CAD build for the part. Positions are in the model's coordinates, mm. Face numbers are marked on the shaded views. A direction names the side the tool comes from. Give positions to 0.01 mm unless a question says otherwise; leave off trailing zeros. Loops run counter-clockwise (first coordinate to the right, second up) from the corner with the lowest first, then second, coordinate; pieces in that order, holes last. Notation, with made-up numbers: (36.25, 85) - (90.25, 85) arc R26 ccw to (90.25, 102) - close; hole circle Ø10 at (-11, 87). An arc over 180 degrees is marked (long way). Return JSON: item names as keys, results as strings.
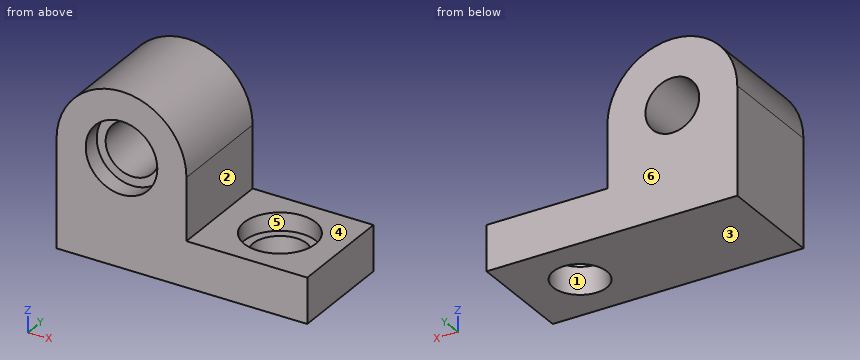
from build123d import *

# Parameters (mm, degrees)
F0_R     = 25.4
F0_R_2   = 19.05
F1_DEPTH = 76.2
F2_DEPTH = 12.7
F3_R     = 19.05
F4_DEPTH = 32.133529
F3_R_2   = 25.4
F5_DEPTH = 12.7


with BuildPart() as f1:
    # F0 (on Front) → F1 (new body)
    with BuildSketch(Plane.XZ):
        with BuildLine():
            Line((0, 76.2), (0, 0))
            Line((0, 0), (177.8, 0))
            Line((177.8, 0), (177.8, 32.132529))
            Line((177.8, 32.132529), (92.11325, 32.132529))
            Line((92.11325, 32.132529), (92.11325, 76.2))
            ThreePointArc((92.11325, 76.2), (46.056625, 122.256625), (0, 76.2))
        make_face()
        with Locations((46.056625, 76.2)):
            Circle(F0_R, mode=Mode.SUBTRACT)
        with Locations((46.056625, 76.2)):
            Circle(F0_R)
        with Locations((46.056625, 76.2)):
            Circle(F0_R_2, mode=Mode.SUBTRACT)
    extrude(amount=-F1_DEPTH)

    # F0 (on Front) → F2 (cut)
    with BuildSketch(Plane.XZ):
        with Locations((46.056625, 76.2)):
            Circle(F0_R)
        with Locations((46.056625, 76.2)):
            Circle(F0_R_2, mode=Mode.SUBTRACT)
    extrude(amount=-F2_DEPTH, mode=Mode.SUBTRACT)

    # F3 (on face) → F4 (cut, through all)
    with BuildSketch(Plane.XY.offset(32.132529)):
        with Locations((134.956625, 38.1)):
            Circle(F3_R)
    extrude(amount=-F4_DEPTH, mode=Mode.SUBTRACT)

    # F3 (on face) → F5 (cut)
    with BuildSketch(Plane.XY.offset(32.132529)):
        with Locations((134.956625, 38.1)):
            Circle(F3_R_2)
        with Locations((134.956625, 38.1)):
            Circle(F3_R, mode=Mode.SUBTRACT)
    extrude(amount=-F5_DEPTH, mode=Mode.SUBTRACT)


solid = f1.part
1. Pull direction X, two halves, no side cores. Call the marked faces 1, 2 and 3: +X half, -X half, draft (parallel to the pull), parting line (faces both ways), or undercut.
Values follow:
{"face 1": "undercut", "face 2": "+X half", "face 3": "draft"}
2. Cut at B-B, the plane x = 123. Write the cut outline in (y, z), plus the area to 3 significant figures.
Values follow:
{"outline": "(0, 0) - (23.27, 0) - (23.27, 19.43) - (15.69, 19.43) - (15.69, 32.13) - (0, 32.13) - close; (52.93, 0) - (76.2, 0) - (76.2, 32.13) - (60.51, 32.13) - (60.51, 19.43) - (52.93, 19.43) - close", "area": "1,300 mm²"}
3. Cut at D-D, the plane z = 63.5. Write the cut outline in (x, y).
Values follow:
{"outline": "(0, 0) - (24.06, 0) - (24.06, 12.7) - (31.86, 12.7) - (31.86, 76.2) - (0, 76.2) - close; (60.26, 12.7) - (68.05, 12.7) - (68.05, 0) - (92.11, 0) - (92.11, 76.2) - (60.26, 76.2) - close"}
4. Drill centre lines: probe 1 along X at (y, z) = (69, 75.5); probe 2 along Z at (x, y) = (45, 5); probe 3 along Z at (x, y) = (119, 23). Where is each one in solid material? Low to high.
Values follow:
{"probe 1": "x = 0 to 27.02, 65.09 to 92.11", "probe 2": "z = 0 to 50.82, 101.58 to 122.24", "probe 3": "z = 0 to 19.43"}
5. Drop flat-ended pins along their axis: P1, Ø1.5, axis at x = 58, z = 88, coming from the +Y side; P2, Ø1.5, axis at y = 14.5, z = 58.5, coming from the +X side; P3, Ø1, axis at y = 59, z = 106, coming from the -X side; P4, Ø2, axis at x = 25, y = 47.5, coming from the +Z side. Give the stop position or say it passes through.
Values follow:
{"P1": "passes through", "P2": "stops at x = 92.11", "P3": "stops at x = 10.52", "P4": "stops at z = 117.66"}
6. Which spindle directions (+Z, -Z, +X, -X, +Y, -Y) get a long thin tool onto all of the face, cutting with end or side? Do the marked faces 4, 5 and 6. Say none if no direction does.
Values follow:
{"face 4": "+Z, +X, +Y, -Y", "face 5": "+Z", "face 6": "+Z, -Z, +X, -X, +Y"}
